Geometry check sheet. Reference: the model listing, model coordinates, mm. Give positions to 0.01 mm unless a question says otherwise; leave off trailing zeros. Loops run counter-clockwise (first coordinate to the right, second up) from the corner with the lowest first, then second, coordinate; pieces in that order, holes last. Notation, with made-up numbers: (-37.5, 25.25) -> (-8.5, 25.25) arc R18 cw to (-8.5, 29.25) -> close; hole circle Ø5 at (22, -30.75). An arc over 180 degrees is marked (long way). Write item = value, one per line. Start each with the question number.
```python
from build123d import *

# Parameters (mm, degrees)
EXTRUDE_1_DEPTH     = 6
SKETCH_2_W          = 150
SKETCH_2_H          = 10
CUT_EXTRUDE_1_DEPTH = 2
FILLET_3_R          = 2
SKETCH_3_W          = 47
SKETCH_3_H          = 6
CUT_EXTRUDE_2_DEPTH = 1
HOLE_WIZARD_M31_D   = 3.4
CUT_EXTRUDE_3_DEPTH = 112.937482552
CUT_EXTRUDE_4_REACH = 114.027
FILLET_1_R          = 2


with BuildPart() as part:
    # Эскиз1 → Бобышка-Вытянуть1 (new body)
    with BuildSketch(Plane(origin=(0, 0, 0), x_dir=(1, 0, 0), z_dir=(0, 1, 0))):
        Polygon((-22.5, 3), (22.5, 3), (22.5, -3), (75, -63), (75, -83), (-75, -83), (-75, -63), (-22.5, -3), align=None)
    extrude(amount=EXTRUDE_1_DEPTH)

    # Эскиз2 → Вырез-Вытянуть1 (cut)
    with BuildSketch(Plane(origin=(0, 6, 0), x_dir=(1, 0, 0), z_dir=(0, 1, 0))):
        with Locations((0, -73)):
            Rectangle(SKETCH_2_W, SKETCH_2_H)
    extrude(amount=-CUT_EXTRUDE_1_DEPTH, mode=Mode.SUBTRACT)

    # Скругление3
    fillet_3_edges = [part.edges().sort_by_distance(p)[0] for p in [
        (-22.5, 3, 3),
        (22.5, 3, 3),
    ]]
    fillet(fillet_3_edges, radius=FILLET_3_R)

    # Эскиз3 → Вырез-Вытянуть2 (cut)
    with BuildSketch(Plane(origin=(0, 6, 0), x_dir=(1, 0, 0), z_dir=(0, 1, 0))):
        Rectangle(SKETCH_3_W, SKETCH_3_H)
    extrude(amount=-CUT_EXTRUDE_2_DEPTH, mode=Mode.SUBTRACT)

    # Отверстие с зазором M31 (through all)
    with Locations(Plane(origin=(0, 0, 0), x_dir=(-1, 0, 0), z_dir=(0, -1, 0))):
        with Locations((-13.5, 0), (-4.5, 0), (4.5, 0), (13.5, 0)):
            Hole(HOLE_WIZARD_M31_D / 2)

    # Эскиз9 → Вырез-Вытянуть3 (cut, through all)
    with BuildSketch(Plane(origin=(0, 4, 0), x_dir=(1, 0, 0), z_dir=(0, 1, 0))):
        with BuildLine():
            Line((-60, -71.4), (60, -71.4))
            ThreePointArc((60, -71.4), (61.6, -73), (60, -74.6))
            Line((60, -74.6), (-60, -74.6))
            ThreePointArc((-60, -74.6), (-61.6, -73), (-60, -71.4))
        make_face()
    extrude(amount=-CUT_EXTRUDE_3_DEPTH, mode=Mode.SUBTRACT)

    # Эскиз10 → Вырез-Вытянуть4 (cut, up to next)
    with BuildSketch(Plane(origin=(0, 6, 0), x_dir=(1, 0, 0), z_dir=(0, 1, 0)), mode=Mode.PRIVATE) as cut_extrude_4_sk1:
        Polygon((-70.559927094, -64), (-56.559927094, -48), (-42.559927094, -64), align=None)
    cut_extrude_4_tool1 = extrude(cut_extrude_4_sk1.sketch, amount=-CUT_EXTRUDE_4_REACH, mode=Mode.PRIVATE) & part.part
    # Эскиз10 → Вырез-Вытянуть4 (cut, up to next)
    with BuildSketch(Plane(origin=(0, 6, 0), x_dir=(1, 0, 0), z_dir=(0, 1, 0)), mode=Mode.PRIVATE) as cut_extrude_4_sk2:
        Polygon((-51.709923067, -48), (-37.709923067, -64), (-23.709923067, -48), align=None)
    cut_extrude_4_tool2 = extrude(cut_extrude_4_sk2.sketch, amount=-CUT_EXTRUDE_4_REACH, mode=Mode.PRIVATE) & part.part
    # Эскиз10 → Вырез-Вытянуть4 (cut, up to next)
    with BuildSketch(Plane(origin=(0, 6, 0), x_dir=(1, 0, 0), z_dir=(0, 1, 0)), mode=Mode.PRIVATE) as cut_extrude_4_sk3:
        Polygon((-18.85991904, -48), (-32.85991904, -64), (-4.85991904, -64), align=None)
    cut_extrude_4_tool3 = extrude(cut_extrude_4_sk3.sketch, amount=-CUT_EXTRUDE_4_REACH, mode=Mode.PRIVATE) & part.part
    # Эскиз10 → Вырез-Вытянуть4 (cut, up to next)
    with BuildSketch(Plane(origin=(0, 6, 0), x_dir=(1, 0, 0), z_dir=(0, 1, 0)), mode=Mode.PRIVATE) as cut_extrude_4_sk4:
        Polygon((-14.009915012, -48), (-0.009915012, -64), (13.990084988, -48), align=None)
    cut_extrude_4_tool4 = extrude(cut_extrude_4_sk4.sketch, amount=-CUT_EXTRUDE_4_REACH, mode=Mode.PRIVATE) & part.part
    # Эскиз10 → Вырез-Вытянуть4 (cut, up to next)
    with BuildSketch(Plane(origin=(0, 6, 0), x_dir=(1, 0, 0), z_dir=(0, 1, 0)), mode=Mode.PRIVATE) as cut_extrude_4_sk5:
        Polygon((18.840089015, -48), (4.840089015, -64), (32.840089015, -64), align=None)
    cut_extrude_4_tool5 = extrude(cut_extrude_4_sk5.sketch, amount=-CUT_EXTRUDE_4_REACH, mode=Mode.PRIVATE) & part.part
    # Эскиз10 → Вырез-Вытянуть4 (cut, up to next)
    with BuildSketch(Plane(origin=(0, 6, 0), x_dir=(1, 0, 0), z_dir=(0, 1, 0)), mode=Mode.PRIVATE) as cut_extrude_4_sk6:
        Polygon((23.690093042, -48), (37.690093042, -64), (51.690093042, -48), align=None)
    cut_extrude_4_tool6 = extrude(cut_extrude_4_sk6.sketch, amount=-CUT_EXTRUDE_4_REACH, mode=Mode.PRIVATE) & part.part
    # Эскиз10 → Вырез-Вытянуть4 (cut, up to next)
    with BuildSketch(Plane(origin=(0, 6, 0), x_dir=(1, 0, 0), z_dir=(0, 1, 0)), mode=Mode.PRIVATE) as cut_extrude_4_sk7:
        Polygon((42.540097069, -64), (70.540097069, -64), (56.540097069, -48), align=None)
    cut_extrude_4_tool7 = extrude(cut_extrude_4_sk7.sketch, amount=-CUT_EXTRUDE_4_REACH, mode=Mode.PRIVATE) & part.part
    # Эскиз10 → Вырез-Вытянуть4 (cut, up to next)
    with BuildSketch(Plane(origin=(0, 6, 0), x_dir=(1, 0, 0), z_dir=(0, 1, 0)), mode=Mode.PRIVATE) as cut_extrude_4_sk8:
        Polygon((-53.059927094, -44), (-39.059927094, -28), (-25.059927094, -44), align=None)
    cut_extrude_4_tool8 = extrude(cut_extrude_4_sk8.sketch, amount=-CUT_EXTRUDE_4_REACH, mode=Mode.PRIVATE) & part.part
    # Эскиз10 → Вырез-Вытянуть4 (cut, up to next)
    with BuildSketch(Plane(origin=(0, 6, 0), x_dir=(1, 0, 0), z_dir=(0, 1, 0)), mode=Mode.PRIVATE) as cut_extrude_4_sk9:
        Polygon((-33.545538953, -28), (-19.545538953, -44), (-5.545538953, -28), align=None)
    cut_extrude_4_tool9 = extrude(cut_extrude_4_sk9.sketch, amount=-CUT_EXTRUDE_4_REACH, mode=Mode.PRIVATE) & part.part
    # Эскиз10 → Вырез-Вытянуть4 (cut, up to next)
    with BuildSketch(Plane(origin=(0, 6, 0), x_dir=(1, 0, 0), z_dir=(0, 1, 0)), mode=Mode.PRIVATE) as cut_extrude_4_sk10:
        Polygon((-0.031150813, -28), (-14.031150813, -44), (13.968849187, -44), align=None)
    cut_extrude_4_tool10 = extrude(cut_extrude_4_sk10.sketch, amount=-CUT_EXTRUDE_4_REACH, mode=Mode.PRIVATE) & part.part
    # Эскиз10 → Вырез-Вытянуть4 (cut, up to next)
    with BuildSketch(Plane(origin=(0, 6, 0), x_dir=(1, 0, 0), z_dir=(0, 1, 0)), mode=Mode.PRIVATE) as cut_extrude_4_sk11:
        Polygon((5.483237327, -28), (19.483237327, -44), (33.483237327, -28), align=None)
    cut_extrude_4_tool11 = extrude(cut_extrude_4_sk11.sketch, amount=-CUT_EXTRUDE_4_REACH, mode=Mode.PRIVATE) & part.part
    # Эскиз10 → Вырез-Вытянуть4 (cut, up to next)
    with BuildSketch(Plane(origin=(0, 6, 0), x_dir=(1, 0, 0), z_dir=(0, 1, 0)), mode=Mode.PRIVATE) as cut_extrude_4_sk12:
        Polygon((24.997625468, -44), (38.997625468, -28), (52.997625468, -44), align=None)
    cut_extrude_4_tool12 = extrude(cut_extrude_4_sk12.sketch, amount=-CUT_EXTRUDE_4_REACH, mode=Mode.PRIVATE) & part.part
    # Эскиз10 → Вырез-Вытянуть4 (cut, up to next)
    with BuildSketch(Plane(origin=(0, 6, 0), x_dir=(1, 0, 0), z_dir=(0, 1, 0)), mode=Mode.PRIVATE) as cut_extrude_4_sk13:
        Polygon((-35.559927094, -24), (-20.684927094, -7), (-5.809927094, -24), align=None)
    cut_extrude_4_tool13 = extrude(cut_extrude_4_sk13.sketch, amount=-CUT_EXTRUDE_4_REACH, mode=Mode.PRIVATE) & part.part
    # Эскиз10 → Вырез-Вытянуть4 (cut, up to next)
    with BuildSketch(Plane(origin=(0, 6, 0), x_dir=(1, 0, 0), z_dir=(0, 1, 0)), mode=Mode.PRIVATE) as cut_extrude_4_sk14:
        Polygon((-14.904785308, -7), (-0.029785308, -24), (14.845214692, -7), align=None)
    cut_extrude_4_tool14 = extrude(cut_extrude_4_sk14.sketch, amount=-CUT_EXTRUDE_4_REACH, mode=Mode.PRIVATE) & part.part
    # Эскиз10 → Вырез-Вытянуть4 (cut, up to next)
    with BuildSketch(Plane(origin=(0, 6, 0), x_dir=(1, 0, 0), z_dir=(0, 1, 0)), mode=Mode.PRIVATE) as cut_extrude_4_sk15:
        Polygon((20.625356478, -7), (5.750356478, -24), (35.500356478, -24), align=None)
    cut_extrude_4_tool15 = extrude(cut_extrude_4_sk15.sketch, amount=-CUT_EXTRUDE_4_REACH, mode=Mode.PRIVATE) & part.part
    add(cut_extrude_4_tool1.solids().sort_by_distance((-56.559927, 6, 58.666667))[0], mode=Mode.SUBTRACT)
    add(cut_extrude_4_tool2.solids().sort_by_distance((-37.709923, 6, 53.333333))[0], mode=Mode.SUBTRACT)
    add(cut_extrude_4_tool3.solids().sort_by_distance((-18.859919, 6, 58.666667))[0], mode=Mode.SUBTRACT)
    add(cut_extrude_4_tool4.solids().sort_by_distance((-0.009915, 6, 53.333333))[0], mode=Mode.SUBTRACT)
    add(cut_extrude_4_tool5.solids().sort_by_distance((18.840089, 6, 58.666667))[0], mode=Mode.SUBTRACT)
    add(cut_extrude_4_tool6.solids().sort_by_distance((37.690093, 6, 53.333333))[0], mode=Mode.SUBTRACT)
    add(cut_extrude_4_tool7.solids().sort_by_distance((56.540097, 6, 58.666667))[0], mode=Mode.SUBTRACT)
    add(cut_extrude_4_tool8.solids().sort_by_distance((-39.059927, 6, 38.666667))[0], mode=Mode.SUBTRACT)
    add(cut_extrude_4_tool9.solids().sort_by_distance((-19.545539, 6, 33.333333))[0], mode=Mode.SUBTRACT)
    add(cut_extrude_4_tool10.solids().sort_by_distance((-0.031151, 6, 38.666667))[0], mode=Mode.SUBTRACT)
    add(cut_extrude_4_tool11.solids().sort_by_distance((19.483237, 6, 33.333333))[0], mode=Mode.SUBTRACT)
    add(cut_extrude_4_tool12.solids().sort_by_distance((38.997625, 6, 38.666667))[0], mode=Mode.SUBTRACT)
    add(cut_extrude_4_tool13.solids().sort_by_distance((-20.684927, 6, 18.333333))[0], mode=Mode.SUBTRACT)
    add(cut_extrude_4_tool14.solids().sort_by_distance((-0.029785, 6, 12.666667))[0], mode=Mode.SUBTRACT)
    add(cut_extrude_4_tool15.solids().sort_by_distance((20.625356, 6, 18.333333))[0], mode=Mode.SUBTRACT)

    # Скругление1
    fillet_1_edges = [part.edges().sort_by_distance(p)[0] for p in [
        (-42.559927094, 3, 64),
        (-70.559927094, 3, 64),
        (-56.559927094, 3, 48),
        (-51.709923067, 3, 48),
        (-23.709923067, 3, 48),
        (-37.709923067, 3, 64),
        (75, 3, 63),
        (75, 3, 83),
        (-75, 3, 83),
        (-75, 3, 63),
        (-18.85991904, 3, 48),
        (-4.85991904, 3, 64),
        (-32.85991904, 3, 64),
        (-14.009915012, 3, 48),
        (13.990084988, 3, 48),
        (-0.009915012, 3, 64),
        (18.840089015, 3, 48),
        (32.840089015, 3, 64),
        (4.840089015, 3, 64),
        (23.690093042, 3, 48),
        (51.690093042, 3, 48),
        (37.690093042, 3, 64),
        (-25.059927094, 3, 44),
        (-53.059927094, 3, 44),
        (-39.059927094, 3, 28),
        (42.540097069, 3, 64),
        (56.540097069, 3, 48),
        (70.540097069, 3, 64),
        (-33.545538953, 3, 28),
        (-5.545538953, 3, 28),
        (-19.545538953, 3, 44),
        (-0.031150813, 3, 28),
        (13.968849187, 3, 44),
        (-14.031150813, 3, 44),
        (5.483237327, 3, 28),
        (33.483237327, 3, 28),
        (19.483237327, 3, 44),
        (52.997625468, 3, 44),
        (24.997625468, 3, 44),
        (38.997625468, 3, 28),
        (-5.809927094, 3, 24),
        (-35.559927094, 3, 24),
        (-20.684927094, 3, 7),
        (-14.904785308, 3, 7),
        (14.845214692, 3, 7),
        (-0.029785308, 3, 24),
        (20.625356478, 3, 7),
        (35.500356478, 3, 24),
        (5.750356478, 3, 24),
    ]]
    fillet(fillet_1_edges, radius=FILLET_1_R)


solid = part.part
```
1) Section check B-B (x = 4.5). Give the number of separate pieces and of enclosed holes in the cut face, plus the area to 3 significant figures.
2) Section check C-C (z = 38). Enter the section's corners in (x, y) (3 decimals), plus the area to 4 significant figures.
3) Depth check by flat-ended pin: pin 1 Ø3 at (y, z) = (3, 7.5) entering from -X; pin 2 Ø0.6 at (x, y) = (21, 5.5) entering from -Z; pin 3 Ø1.8 at (x, y) = (36, 3) entering from -Z; pin 4 Ø3 at (x, z) = (-19, 42.5) entering from -Y. Enter the tip coordinate at first touch or a pass-through.
4) Draft check along Z on faces 1 (the flat face through (-22.5, 2, 0)), 2 (the flat face through (-6.4, 3, 56.7)). Enter one of: released by +Z, released by -Z, zero draft, split by the parting line, or undercut.
5) Thickness scan on line 1 (Z direction, x = 22, y = 3.75); line 2 (Z direction, x = -42, y = 1); line 3 (Z direction, x = -46, y = 2). Record the ranges inside material, lowest first.
6) Section check A-A (z = 73). Enter the section's corners in (x, y).
Check result:
q1.separate_pieces = 6
q1.enclosed_holes = 0
q1.area = 259 mm2
q2.outline = (-53.125, 0) -> (-47.81, 0) -> (-47.81, 6) -> (-53.125, 6) -> close; (-30.31, 0) -> (-24.796, 0) -> (-24.796, 6) -> (-30.31, 6) -> close; (-14.296, 0) -> (-8.781, 0) -> (-8.781, 6) -> (-14.296, 6) -> close; (8.719, 0) -> (14.233, 0) -> (14.233, 6) -> (8.719, 6) -> close; (24.733, 0) -> (30.248, 0) -> (30.248, 6) -> (24.733, 6) -> close; (47.748, 0) -> (53.125, 0) -> (53.125, 6) -> (47.748, 6) -> close
q2.area = 196.5 mm2
q3.pin_1 = -27.75
q3.pin_2 = 3
q3.pin_3 = 17.4
q3.pin_4 = 0
q4.face_1 = zero draft
q4.face_2 = undercut
q5.line_1 = -3 to 8.58, 24 to 28, 41.12 to 51.61, 64 to 71.4, 74.6 to 83
q5.line_2 = 25.29 to 31.36, 44 to 48, 59.1 to 71.4, 74.6 to 83
q5.line_3 = 29.86 to 35.93, 44 to 48, 54.53 to 60.07, 63.75 to 71.4, 74.6 to 83
q6.outline = (-75, 0) -> (-61.6, 0) -> (-61.6, 4) -> (-75, 4) -> close; (61.6, 0) -> (75, 0) -> (75, 4) -> (61.6, 4) -> close
